Design review of the part built by this model. Coordinates are the model's own, in mm. Face numbers are marked on the shaded views. Coordinates: 2 decimals unless noted, no trailing zeros. Loops run counter-clockwise (first coordinate to the right, second up) from the corner with the lowest first, then second, coordinate; pieces in that order, holes last.
Q1. Add section D-D on y = 32.5. Give the boundary of the cut face in (x, z).
Q2. Wall thickness on probe 1 along X at (y, z) = (6, 1); probe 2 along X at (y, z) = (42, 7); probe 3 along Z at (x, y) = (37.5, 20): over which ranges is each line inside the solid? List them lowest first.
Q3. Draft analysis for pull direction X (two halves, no side actions). For the marked faces 1, 2 and 3, state which applies: released by +X, released by -X, zero draft, split by the parting line, or undercut.
Q4. Add section A-A on y = -14.5. Give the boundary of the cut face in (x, z).
Q5. Add section B-B on z = 26.5. Give the boundary of the cut face in (x, y).
Q6. For P1, Ø4.5, axis at x = 26.99, y = 6.35, coming from the +Z side; P2, Ø5, axis at x = -23, z = 37.5, coming from the -Y side; P3, Ø3, axis at x = -26.99, y = 6.35, coming from the -Z side, all flat-tipped, find the tip position at first contact; note any pin that passes through.
Q7. Add section C-C on x = -37.5. Give the boundary of the cut face in (y, z), and give its area (3 significant figures).
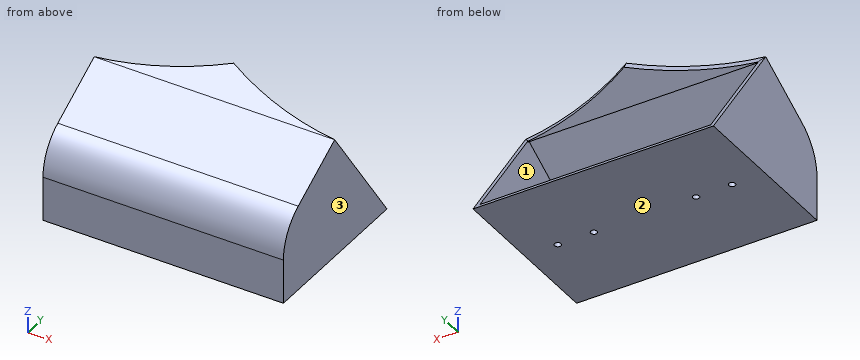
```python
from build123d import *

# Parameters (mm, degrees)
BOSS_EXTRUDE1_DEPTH = 63.5
FILLET1_R           = 25.4
SHELL1_T            = -2.54
BOSS_EXTRUDE4_DEPTH = 3.81
CUT_EXTRUDE2_REACH  = 75.025
SKETCH6_R           = 1.6891


with BuildPart() as part:
    # Sketch2 → Boss-Extrude1 (new body, symmetric)
    with BuildSketch(Plane(origin=(0, 0, 0), x_dir=(0, 0, -1), z_dir=(1, 0, 0))):
        Polygon((0, 50.8), (0, -38.1), (-38.1, -38.1), (-63.5, 5.894090512), align=None)
    extrude(amount=BOSS_EXTRUDE1_DEPTH, both=True)

    # Fillet1
    fillet1_edges = [part.edges().sort_by_distance(p)[0] for p in [
        (0, -38.1, 38.1),
    ]]
    fillet(fillet1_edges, radius=FILLET1_R)

    # Shell1
    shell1_openings = [part.faces().sort_by_distance(p)[0] for p in [
        (0, 28.347045256, 31.75),
    ]]
    offset(amount=SHELL1_T, openings=shell1_openings, kind=Kind.INTERSECTION)

    # Sketch3 → Boss-Extrude4 (add)
    with BuildSketch(Plane(origin=(0, -26.022783942, 45.072783942), x_dir=(1, 0, 0), z_dir=(0, -0.5, 0.866025404))):
        with BuildLine():
            Line((-63.5, 36.854432116), (63.5, 36.854432116))
            ThreePointArc((63.5, 36.854432116), (30.854255532, 43.393617223), (0, 55.904432116))
            ThreePointArc((0, 55.904432116), (-30.854255532, 43.393617223), (-63.5, 36.854432116))
        make_face()
    extrude(amount=-BOSS_EXTRUDE4_DEPTH)

    # Sketch6 → Cut-Extrude2 (cut, up to next)
    with BuildSketch(Plane(origin=(0, 0, 0), x_dir=(-1, 0, 0), z_dir=(0, 0, -1)), mode=Mode.PRIVATE) as cut_extrude2_sk1:
        with Locations((-46.0375, 6.35)):
            Circle(SKETCH6_R)
    cut_extrude2_tool1 = extrude(cut_extrude2_sk1.sketch, amount=-CUT_EXTRUDE2_REACH, mode=Mode.PRIVATE) & part.part
    add(cut_extrude2_tool1.solids().sort_by_distance((46.0375, 6.35, 0))[0], mode=Mode.SUBTRACT)
    # Sketch6 → Cut-Extrude2 (cut, up to next)
    with BuildSketch(Plane(origin=(0, 0, 0), x_dir=(-1, 0, 0), z_dir=(0, 0, -1)), mode=Mode.PRIVATE) as cut_extrude2_sk2:
        with Locations((-26.9875, 6.35)):
            Circle(SKETCH6_R)
    cut_extrude2_tool2 = extrude(cut_extrude2_sk2.sketch, amount=-CUT_EXTRUDE2_REACH, mode=Mode.PRIVATE) & part.part
    add(cut_extrude2_tool2.solids().sort_by_distance((26.9875, 6.35, 0))[0], mode=Mode.SUBTRACT)
    # Sketch6 → Cut-Extrude2 (cut, up to next)
    with BuildSketch(Plane(origin=(0, 0, 0), x_dir=(-1, 0, 0), z_dir=(0, 0, -1)), mode=Mode.PRIVATE) as cut_extrude2_sk3:
        with Locations((26.9875, 6.35)):
            Circle(SKETCH6_R)
    cut_extrude2_tool3 = extrude(cut_extrude2_sk3.sketch, amount=-CUT_EXTRUDE2_REACH, mode=Mode.PRIVATE) & part.part
    add(cut_extrude2_tool3.solids().sort_by_distance((-26.9875, 6.35, 0))[0], mode=Mode.SUBTRACT)
    # Sketch6 → Cut-Extrude2 (cut, up to next)
    with BuildSketch(Plane(origin=(0, 0, 0), x_dir=(-1, 0, 0), z_dir=(0, 0, -1)), mode=Mode.PRIVATE) as cut_extrude2_sk4:
        with Locations((46.0375, 6.35)):
            Circle(SKETCH6_R)
    cut_extrude2_tool4 = extrude(cut_extrude2_sk4.sketch, amount=-CUT_EXTRUDE2_REACH, mode=Mode.PRIVATE) & part.part
    add(cut_extrude2_tool4.solids().sort_by_distance((-46.0375, 6.35, 0))[0], mode=Mode.SUBTRACT)


solid = part.part
```
Entries:
1. outline: (-63.5, 0) - (63.5, 0) - (63.5, 25.88) - (60.96, 25.88) - (60.96, 2.54) - (-60.96, 2.54) - (-60.96, 25.88) - (-63.5, 25.88) - close
2. probe 1: x = -63.5 to -47.69, -44.39 to -28.64, -25.34 to 25.34, 28.64 to 44.39, 47.69 to 63.5
2. probe 2: x = -63.5 to -60.96, 60.96 to 63.5
2. probe 3: z = 0 to 2.54
3. face 1: undercut
3. face 2: zero draft
3. face 3: released by +X
4. outline: (-63.5, 0) - (63.5, 0) - (63.5, 51.73) - (-63.5, 51.73) - close; hole (-60.96, 2.54) - (60.96, 2.54) - (60.96, 48.79) - (-60.96, 48.79) - close
5. outline: (-63.5, -37.91) - (63.5, -37.91) - (63.5, 32.06) - (60.96, 32.06) - (60.96, -35.35) - (-60.96, -35.35) - (-60.96, 32.06) - (-63.5, 32.06) - close
6. P1: stops at z = 65.06
6. P2: stops at y = -35.31
6. P3: stops at z = 59.96
7. outline: (-38.1, 0) - (50.8, 0) - (49, 2.54) - (-35.56, 2.54) - (-35.56, 23.44) arc R22.86 cw to (-24.13, 43.23) - (7.16, 61.3) - (7.8, 60.2) - (11.86, 62.54) - (9.95, 65.84) - (-25.4, 45.43) arc R25.4 ccw to (-38.1, 23.44) - close
7. area: 450 mm2
